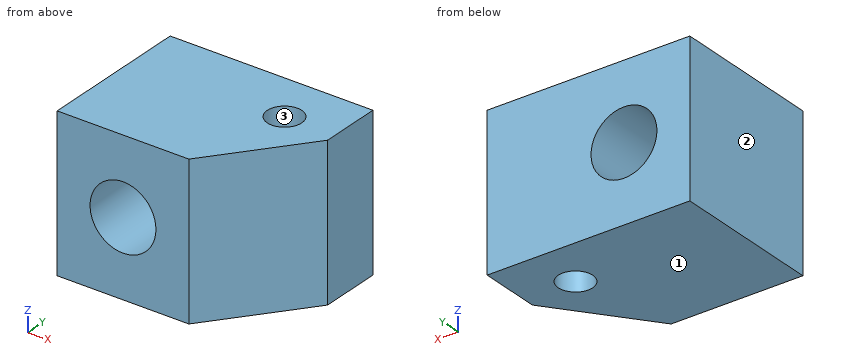
from build123d import *

# Parameters (mm, degrees)
ESTRUSIONE_ESTRUSIONE1_DEPTH = 15
FORO_PER_VITE_M3_1_D         = 3.4
SCHIZZO5_R                   = 3.25
TAGLIO_ESTRUSIONE1_DEPTH     = 25.879710609


with BuildPart() as part:
    # Schizzo1 → Estrusione-Estrusione1 (new body)
    with BuildSketch(Plane.XY):
        Polygon((0, 0), (-13, 0), (-13, 15), (7, 15), (7, 9), align=None)
    extrude(amount=ESTRUSIONE_ESTRUSIONE1_DEPTH)

    # Foro per Vite M3-1 (through all)
    with Locations(Plane.XY.offset(15)):
        with Locations((2, 10)):
            Hole(FORO_PER_VITE_M3_1_D / 2)

    # Schizzo5 → Taglio-Estrusione1 (cut, through all)
    with BuildSketch(Plane(origin=(0, 0, 0), x_dir=(-1, 0, 0), z_dir=(0, -1, 0))):
        with Locations(Location((6.5, -7.5, 0), (0, 0, 180))):
            Circle(SCHIZZO5_R)
    extrude(amount=-TAGLIO_ESTRUSIONE1_DEPTH, mode=Mode.SUBTRACT)


solid = part.part
Geometry check sheet. Reference: the model listing, model coordinates, mm. Face numbers are marked on the shaded views. Give positions to 0.01 mm unless a question says otherwise; leave off trailing zeros. Order: outer loops, then holes, each group sorted by start corner. A loop starts at its lowest first (then second) coordinate and runs counter-clockwise, first axis right, second up.
1. Sectioned sample at D-D (z = 11.25). Record the boundary of the cut face in (x, y), then the cut area to 3 significant figures.
Completed:
outline: (-13, 0) - (0, 0) - (7, 9) - (7, 15) - (-13, 15) - close; hole circle Ø3.4 at (2, 10)
area: 259 mm2
2. Draft check along X on the marked faces 1, 2 and 3. Enter one of: pulls with the +X half, pulls with the -X half, needs draft (parallel to the pull), parting line crosses it, or undercut.
Completed:
face 1: needs draft
face 2: pulls with the -X half
face 3: undercut
3. Sectioned sample at B-B (z = 7.5). Record the boundary of the cut face in (x, y), then the cut area to 3 significant figures.
Completed:
outline: (-13, 0) - (-9.75, 0) - (-9.75, 15) - (-13, 15) - close; (-3.25, 0) - (0, 0) - (7, 9) - (7, 15) - (-3.25, 15) - close; hole circle Ø3.4 at (2, 10)
area: 162 mm2
4. Scan lines: line 1 (Z direction, x = -6.5, y = 5.25); line 2 (X direction, y = 11, z = 10); line 3 (Z direction, x = -4.5, y = 2). Record each from-to range of solid material in increasing order.
Completed:
line 1: z = 0 to 4.25, 10.75 to 15
line 2: x = -13 to -8.58, -4.42 to 0.63, 3.37 to 7
line 3: z = 0 to 4.94, 10.06 to 15
5. Sectioned sample at C-C (x = -6.5). Record the boundary of the cut face in (y, z).
Completed:
outline: (0, 0) - (15, 0) - (15, 4.25) - (0, 4.25) - close; (0, 10.75) - (15, 10.75) - (15, 15) - (0, 15) - close
6. Depth check by flat-ended pin: pin 1 (6 mm diameter, centred on x = 5, z = 3.5, fed in from -Y); pin 2 (1.5 mm diameter, centred on y = 7.5, z = 6, fed in from +X). Enter the tip coordinate at first touch or a pass-through.
Completed:
pin 1: stops at y = 2.57
pin 2: stops at x = 6.42
7. Sectioned sample at A-A (y = 10). Record the boundary of the cut face in (x, z), then the cut area to 3 significant figures.
Completed:
outline: (-13, 0) - (0.3, 0) - (0.3, 15) - (-13, 15) - close; (3.7, 0) - (7, 0) - (7, 15) - (3.7, 15) - close; hole circle Ø6.5 at (-6.5, 7.5)
area: 216 mm2
